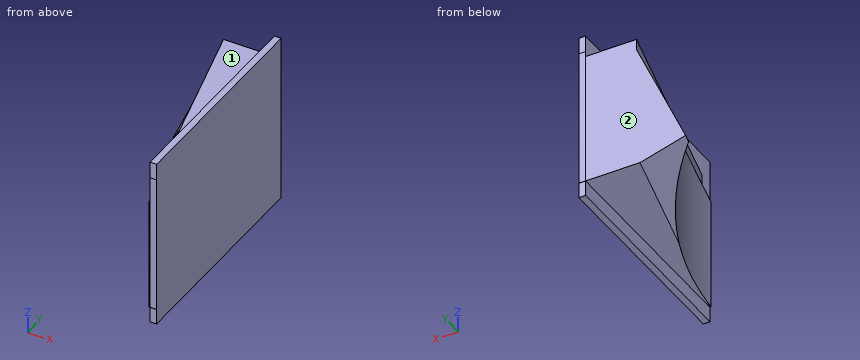
Autodesk Inventor part; units mm, degrees
ref_plane "Work Plane1" through (25.8481, -31.3143, 21.5224) normal (0.9701425, 0.2425356, 0) x (0, 0, -1)
ref_plane "YZ Plane" through (0, 0, 0) normal (1, 0, 0) x (0, 1, 0)
ref_plane "XZ Plane" through (0, 0, 0) normal (0, 1, 0) x (-1, 0, 0)
sketch "Sketch1" plane through (0, 0, 0) normal (0, 0, 1) x (1, 0, 0)
  line L0 (43.3243, -30.319) -> (27.0819, 34.6507)
  line L1 (43.6847, -30.319) -> (43.3243, -30.319)
  line L2 (43.8153, 34.6507) -> (43.6847, -30.319)
  line L3 (27.0819, 34.6507) -> (43.8153, 34.6507)
  point P0 (0, 0)
extrude "Extrusion1" add sketch "Sketch1" along normal blind 40
sketch "Sketch2" plane through (0, 0, 40) normal (0, 0, 1) x (1, 0, 0)
  line L0 (43.6847, -30.319) -> (43.8153, 34.6507)
  line L1 (43.8153, 34.6507) -> (27.0819, 34.6507)
  line L2 (27.0819, 34.6507) -> (43.3243, -30.319)
  line L3 (43.3243, -30.319) -> (43.6847, -30.319)
  line L4 (9.5067, 30.2569) -> (11.5067, 30.2569)
  line L5 (11.5067, 30.2569) -> (11.5067, 34.6507)
  line L6 (11.5067, 34.6507) -> (27.0819, 34.6507)
  line L7 (11.5067, 34.6507) -> (43.3243, -30.319)
  point P0 (0, 0)
  dimension "d2" = 2
extrude "Extrusion2" add sketch "Sketch2" against normal blind 40 contours L7 L6 L2
sketch "Sketch3" plane through (0, 0, 0) normal (0, 0, -1) x (-1, 0, 0)
  line L0 (-43.6847, -30.319) -> (-43.8153, 34.6507)
  line L1 (-43.3243, -30.319) -> (-43.6847, -30.319)
  line L2 (-43.3243, -30.319) -> (-11.5067, 34.6507)
  line L3 (-43.8153, 34.6507) -> (-11.5067, 34.6507)
  arc A0 (-11.5067, 34.6507) -> (-43.3243, -30.319) centre (56.3122, -38.8381) ccw
  point P0 (0, 0)
  dimension "d5" = 100
extrude "Extrusion3" cut sketch "Sketch3" against normal blind 40 contours A0 L2
ref_plane "Work Plane1" through (25.8481, -31.3143, 21.5224) normal (0.9701425, 0.2425356, 0) x (0, 0, -1)
ref_plane "Work Plane4" through (11.5067, 34.6507, 40) normal (0.2425356, -0.9701425, 0) x (0, 0, -1)
ref_plane "Work Plane3" through (25.8481, -31.3143, 21.5224) normal (0.9701425, 0.2425356, 0) x (0, 0, -1)
sketch "Sketch5" plane through (11.5067, 34.6507, 40) normal (0.2425356, -0.9701425, 0) x (0, 0, -1)
  line L0 (29.9641, 1.0219) -> (3.228, 13.4892)
  line L1 (3.228, 13.4892) -> (3.228, 16.4892)
  line L2 (3.228, 16.4892) -> (0, 16.4892)
  line L3 (0, 31.344) -> (0, 0)
  line L4 (40, 31.344) -> (40, 0)
  line L5 (0, 0) -> (40, 0)
  line L6 (0, 31.344) -> (0, 0)
  line L7 (40, 31.344) -> (0, 31.344)
  line L8 (29.9641, 1.0219) -> (40, 1.0219)
  arc A0 (36.6954, 1.9144) -> (36.6283, 1.4007) centre (38.6283, 1.4007) ccw
  line L9 (36.6954, 1.9144) -> (40, 1.9144)
  line L10 (40, 1.9144) -> (40, -5.9625)
  arc A1 (40, -5.9625) -> (38.4823, -3.5717) centre (32.6454, -8.9542) ccw
  arc A2 (36.6283, 1.1737) -> (38.4823, -3.5717) centre (43.6283, 1.1737) ccw
  line L11 (36.6283, 1.1737) -> (36.6283, 1.4007)
  arc A3 (36.867, 2.3482) -> (36.6954, 1.9144) centre (38.6283, 1.4007) ccw
  arc A4 (36.867, 2.3482) -> (40, 14.7848) centre (13.75, 14.7848) ccw
  line L12 (40, 14.7848) -> (40, 31.0187)
  line L13 (44.6283, 31.0187) -> (40, 31.0187)
  line L14 (44.6283, -24.8913) -> (44.6283, 31.0187)
  line L15 (44.6283, -24.8913) -> (40, -24.8913)
  line L16 (40, -24.8913) -> (40, 1.9144)
  line L17 (36.6954, 1.9144) -> (40, 1.9144)
  line L18 (36.6954, 1.9144) -> (3.228, 16.4892)
  line L19 (40, 15.4598) -> (40, 31.344)
  line L20 (40, 14.7848) -> (40, 15.4598)
  line L21 (40, 15.4598) -> (0, 15.4598)
  line L22 (40, 15.4598) -> (36.1857, 2.1363)
  point P0 (40, -19.5671)
  point P1 (0, 0)
  point P2 (36.7274, 0)
  dimension "d10" = 3
extrude "Extrusion4" cut sketch "Sketch5" along normal blind 72.5 contours L8 A2 L5 L3 L21 L1 L0 | L0 L1 L21 L18 A0 L11 A2 L8 | A2 L11 A0 L9 L4 L8 | L8 L4 L5 A2 | L21 L3 L2 L1 | L1 L18 L21 | L5 L10 A1 A2 | L9 A3 A4 L4 | L22 L4 A4 A3 L18
sketch "Sketch6" plane through (43.8153, 34.6507, 40) normal (0.999998, -0.0020114, 0) x (0, 0, -1)
  line L0 (40, -0.0453) -> (40, -65.0151)
  line L1 (44.6283, -65.0151) -> (40, -65.0151)
  line L2 (44.6283, -0.0453) -> (44.6283, -65.0151)
  line L3 (44.6283, -0.0453) -> (40, -0.0453)
  line L4 (-1.673, -64.9698) -> (-6.673, -64.9644)
  line L5 (-1.673, -64.9698) -> (-1.6028, -0.0003)
  line L6 (-6.6028, 0.0051) -> (-1.6028, -0.0003)
  line L7 (-6.673, -64.9644) -> (-6.6028, 0.0051)
  line L8 (0, -60.7594) -> (0, 0)
  line L9 (0, 0) -> (-1.6685, 0)
  line L10 (-1.6685, 0) -> (-1.6685, -60.7144)
  line L11 (-1.6685, -60.7144) -> (0, -60.7144)
  line L12 (0, -60.7144) -> (0, 0)
  line L13 (40, -64.9698) -> (40, 0)
  line L14 (40, 0) -> (0, 0)
  line L15 (0, 0) -> (0, -60.7144)
  line L16 (0, -60.7144) -> (40, -60.7144)
  line L17 (40, -60.7144) -> (40, 0)
  line L18 (40, -64.9698) -> (-1.673, -64.9698)
  point P0 (40, -34.7388)
  point P1 (-1.6685, -0.0002)
  point P2 (40, -60.7144)
extrude "Extrusion5" add sketch "Sketch6" along normal blind 2
properties part number "Lid"
The model under review builds one solid part; all positions refer to its coordinate system, in mm. Face numbers are marked on the shaded views. A direction names the side the tool comes from. Round coordinates to 2 decimals unless told otherwise and drop trailing zeros. Write each loop counter-clockwise with the first axis right and the second up, starting at its lowest first coordinate (ties: lowest second). Pieces come first, ordered by that corner, then holes. Notation, with made-up numbers: M -16.5,88.25 L -4.5,88.25 A15 ccw -4.5,99.25 Z; hole C -3.5,83 d11. An arc over 180 degrees is marked long. Answer as CSV lines item,"result". Start each with the question number.
Q1. Consider section C-C, the plane z = 14. Give the boundary of the cut face in (x, y).
Q2. Consider section B-B, the plane y = 0. Give the boundary of the cut face in (x, z).
Q3. Consider section D-D, the plane y = 9.5. Give the boundary of the cut face in (x, z).
Q4. Tool access review of the marked faces 1 and 2: name each direction out of +Z, -Z, +X, -X, +Y, -Y from which nothing blocks a thin tool from reaching the whole face with its end or side.
Q5. Clearance check with flat-ended pins moving along their axes: P1, Ø12, axis at y = -11, z = 27, coming from the -X side; P2, Ø1, axis at y = -15.5, z = 35.5, coming from the -X side (3 decimals); P3, Ø3, axis at x = 33, y = 11, coming from the +Z side. State where each tip first meets the part, or that it passes through.
Q6. Consider section A-A, the plane x = 32. Give the boundary of the cut face in (y, z), then the cut area to 3 significant figures.
Q7. Wall thickness on line 1 along Z through (x, y) = (35.5, 26); line 2 along X through (y, z) = (-21, 41); line 3 along Z through (x, y) = (44.5, -13): over which ranges is each line inside the solid? List them lowest first.
Result set:
1,outline,"M 18.28,34.65 L 20.71,24.94 A100 cw 43.32,-30.32 L 43.68,-30.32 L 45.68,-30.32 L 45.82,34.65 L 43.82,34.65 Z"
2,outline,"M 35.84,0.07 L 36.1,0 L 43.75,0 L 43.75,-4.63 L 45.75,-4.63 L 45.75,46.64 L 43.75,46.64 L 43.75,40 L 37.17,40 L 37.17,36.77 L 35.84,33.81 Z"
3,outline,"M 31.23,0.69 L 33.73,0 L 43.76,0 L 43.76,-4.63 L 45.76,-4.63 L 45.76,46.63 L 43.76,46.63 L 43.76,40 L 34.79,40 L 34.79,36.77 L 31.23,28.84 Z"
4,face 1,"+Z, -X, +Y, -Y"
4,face 2,"+Z, -Z, +X, -X, +Y"
5,P1,"stops at x = 37.79"
5,P2,"stops at x = 40.805"
5,P3,"stops at z = 40"
6,outline,"M 8.08,0.58 L 16.42,0 L 34.65,0 L 34.65,40 L 20.66,40 L 20.66,36.77 L 8.08,29.76 Z"
6,area,"976 mm²"
7,line 1,"z = 0 to 40"
7,line 2,"x = 43.7 to 45.7"
7,line 3,"z = -4.63 to 46.65"
